The drawing under review shows one solid part. Ordinate dimensions are in mm from its lowest x, y, z. A direction names the side the tool comes from. Give positions to 0.01 mm unless a question says otherwise; leave off trailing zeros. Write each loop counter-clockwise with the first axis right and the second up, starting at its lowest first coordinate (ties: lowest second). Pieces come first, ordered by that corner, then holes. Notation, with made-up numbers: (46, 51.5) -> (79, 51.5) arc R20 ccw to (79, 63.5) -> close; hole circle Ø2 at (36, 28.5). An arc over 180 degrees is marked (long way). Answer as a JSON object with one key per item and string values.
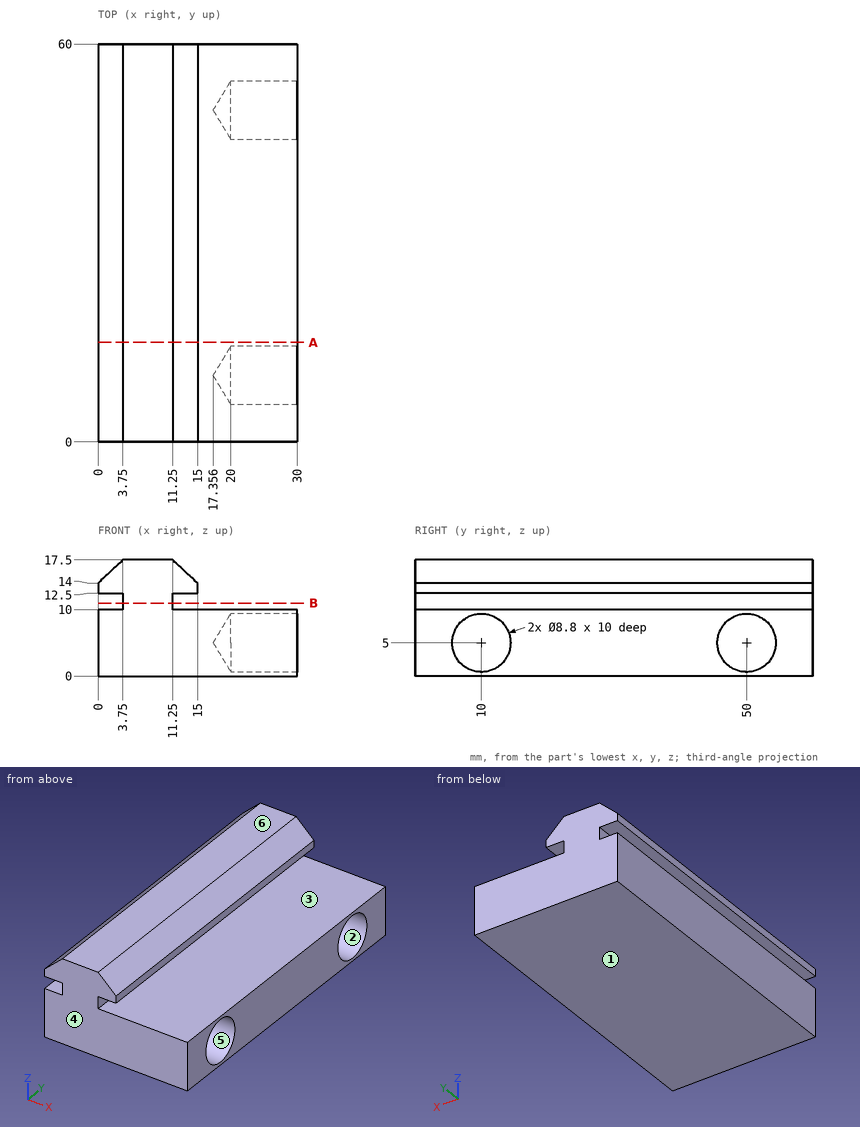
(1) For the marked faces 5 and 6, list the 3-axis set-ups (+Z, -Z, +X, -X, +Y, -Y) from which the entire face can be reached by the end or side of a thin tool; tool diameter is ignored.
Here are the results:
{"face 5": "+X", "face 6": "+Z, +X, -X, +Y, -Y"}
(2) Clearance check with flat-ended pins moving along their axes: pin 1 (1 mm diameter, centred on x = 16.5, z = 11.5, fed in from +Y); pin 2 (1.6 mm diameter, centred on y = 40, z = 13, fed in from +X). State where each tip first meets the part, or that it passes through.
Here are the results:
{"pin 1": "passes through", "pin 2": "stops at x = 15"}
(3) The part is to be moulded in two halves that separate along Z. For the marked faces 1, 2, 3 and 4, say which applies: +Z half, -Z half, draft (parallel to the pull), parting line (faces both ways), or undercut.
Here are the results:
{"face 1": "-Z half", "face 2": "undercut", "face 3": "undercut", "face 4": "draft"}
(4) We need section A-A, the plane y = 15. State the section outline as (x, z) points, then the cut area to 3 significant figures.
Here are the results:
{"outline": "(0, 0) -> (30, 0) -> (30, 10) -> (11.25, 10) -> (11.25, 12.5) -> (15, 12.5) -> (15, 14) -> (11.25, 17.5) -> (3.75, 17.5) -> (0, 14) -> (0, 12.5) -> (3.75, 12.5) -> (3.75, 10) -> (0, 10) -> close", "area": "381 mm²"}
(5) For line 1 along Y through (x, z) = (25, 5); line 2 along Y through (x, z) = (24.5, 1.75) (1 decimal); line 3 along Z through (x, y) = (23.5, 47), list the stretches that pass through material, from the lowest coordinate up.
Here are the results:
{"line 1": "y = 0 to 5.6, 14.4 to 45.6, 54.4 to 60", "line 2": "y = 0 to 7, 13 to 47, 53 to 60", "line 3": "z = 0 to 1.78, 8.22 to 10"}
(6) We need section B-B, the plane z = 11. State the section outline as (x, y) points, then the cut area to 3 significant figures.
Here are the results:
{"outline": "(3.75, 0) -> (11.25, 0) -> (11.25, 60) -> (3.75, 60) -> close", "area": "450 mm²"}
